from build123d import *

# Parameters (mm, degrees)
BOSS_EXTRUDE1_DEPTH       = 2.54
SKETCH2_R                 = 5.08
BOSS_EXTRUDE2_DEPTH       = 6.985
F_6_CLEARANCE_HOLE1_D     = 4.3053
TAP_DRILL_FOR_4_40_TAP1_D = 2.413


with BuildPart() as part:
    # Sketch1 → Boss-Extrude1 (new body)
    with BuildSketch(Plane(origin=(0, 0, 0), x_dir=(1, 0, 0), z_dir=(0, 1, 0))):
        with BuildLine():
            Line((-15.08125, 5.08), (15.08125, 5.08))
            ThreePointArc((15.08125, 5.08), (19.774558025, 1.944031836), (18.673352448, -3.592102448))
            Line((18.673352448, -3.592102448), (3.592102448, -18.673352448))
            ThreePointArc((3.592102448, -18.673352448), (0, -20.16125), (-3.592102448, -18.673352448))
            Line((-3.592102448, -18.673352448), (-18.673352448, -3.592102448))
            ThreePointArc((-18.673352448, -3.592102448), (-19.774558025, 1.944031836), (-15.08125, 5.08))
        make_face()
    extrude(amount=BOSS_EXTRUDE1_DEPTH)

    # Sketch2 → Boss-Extrude2 (add)
    with BuildSketch(Plane.XZ):
        with Locations((-15.08125, 0)):
            Circle(SKETCH2_R)
        with Locations((0, 15.08125)):
            Circle(SKETCH2_R)
        with Locations((15.08125, 0)):
            Circle(SKETCH2_R)
    extrude(amount=BOSS_EXTRUDE2_DEPTH)

    # #6 Clearance Hole1 (through all)
    with Locations(Plane(origin=(0, 2.54, 0), x_dir=(1, 0, 0), z_dir=(0, 1, 0))):
        with Locations((-15.08125, 0), (0, -15.08125), (15.08125, 0)):
            Hole(F_6_CLEARANCE_HOLE1_D / 2)

    # Tap Drill for #4-40 Tap1 (through all)
    with Locations(Plane(origin=(0, 2.54, 0), x_dir=(1, 0, 0), z_dir=(0, 1, 0))):
        with Locations((8.380000004, -2.414999996), (8.380000004, 2.414999996), (-9.650000004, -2.414999996), (-9.650000004, 2.414999996)):
            Hole(TAP_DRILL_FOR_4_40_TAP1_D / 2)


solid = part.part
CAD build for the part. Positions are in the model's coordinates, mm. Coordinates: 2 decimals unless noted, no trailing zeros. Loops run counter-clockwise (first coordinate to the right, second up) from the corner with the lowest first, then second, coordinate; pieces in that order, holes last. Notation, with made-up numbers: (36, 16) -> (87, 16) arc R19 ccw to (87, 44) -> close; hole circle Ø9 at (45, 2). An arc over 180 degrees is marked (long way). One line per item, written item: value.
1. Slice it at B-B on x = 0.5. Write the cut outline in (y, z) (3 decimals).
Answers:
outline: (-6.985, 10.026) -> (0, 10.026) -> (0, -5.08) -> (2.54, -5.08) -> (2.54, 12.987) -> (-6.985, 12.987) -> close; (-6.985, 17.175) -> (2.54, 17.175) -> (2.54, 20.137) -> (-6.985, 20.137) -> close
2. Slice it at D-D on x = 8.38. Write the cut outline in (y, z).
Answers:
outline: (0, -5.08) -> (2.54, -5.08) -> (2.54, -3.62) -> (0, -3.62) -> close; (0, -1.21) -> (2.54, -1.21) -> (2.54, 1.21) -> (0, 1.21) -> close; (0, 3.62) -> (2.54, 3.62) -> (2.54, 13.89) -> (0, 13.89) -> close
3. Slice it at A-A on z = 0. Write the cut outline in (x, y) (3 decimals).
Answers:
outline: (-20.161, -6.985) -> (-17.234, -6.985) -> (-17.234, 2.54) -> (-20.161, 2.54) -> close; (-12.929, -6.985) -> (-10.001, -6.985) -> (-10.001, 0) -> (10.001, 0) -> (10.001, -6.985) -> (12.929, -6.985) -> (12.929, 2.54) -> (-12.929, 2.54) -> close; (17.234, -6.985) -> (20.161, -6.985) -> (20.161, 2.54) -> (17.234, 2.54) -> close
4. Flat gauge pins, fed straight in: P1, Ø5, axis at y = 1, z = 3.5, coming from the +X side; P2, Ø2, axis at x = -3.5, y = -0.5, coming from the +Z side; P3, Ø4, axis at x = -9.65, z = 2.415, coming from the +Y side; P4, Ø4, axis at x = 13.5, y = -1.5, coming from the +Z side. Where does each tip first touch, or does it go through?
Answers:
P1: stops at x = 20.06
P2: stops at z = 19.5
P3: stops at y = 2.54
P4: stops at z = 10.09
5. Pull direction X, two halves, no side cores. Call faces 1 (the face through (16.1, -6.985, -2.2)), 2 (the face through (-11.027, 1.252, 11.238)), 3 (the face through (-10, -3, 0)), 4 (the face through (7.23, 1.25, -2.78)): pulls with the +X half, pulls with the -X half, needs draft (parallel to the pull), parting line crosses it, or undercut.
Answers:
face 1: needs draft
face 2: pulls with the -X half
face 3: undercut
face 4: undercut
6. Drill centre lines: line 1 (Z direction, x = 8.38, y = 1.85); line 2 (X direction, y = -3.25, z = -0.25); line 3 (X direction, y = 1.5, z = -1). Where is each one in solid material? Low to high. Write a range as [from, to].
Answers:
line 1: z = [-5.08, -3.62], [-1.21, 1.21], [3.62, 13.89]
line 2: x = [-20.16, -17.22], [-12.94, -10.01], [10.01, 12.94], [17.22, 20.16]
line 3: x = [-20.06, -16.99], [-13.17, 13.17], [16.99, 20.06]
7. Slice it at C-C on y = -0.5. Give the number of separate pieces and of enclosed holes in the cut face, and give its area (3 significant figures).
Answers:
separate pieces: 3
enclosed holes: 3
area: 199 mm^2
